Model file for the job. Use its own axes, mm. Round coordinates to 2 decimals unless told otherwise and drop trailing zeros. Loops run counter-clockwise (first coordinate to the right, second up) from the corner with the lowest first, then second, coordinate; pieces in that order, holes last.
from build123d import *

# Parameters (mm, degrees)
BOSS_EXTRU_1_DEPTH = 52
CONG_1_R           = 2
ESQUISSE3_R        = 1
BOSS_EXTRU_2_DEPTH = 40


with BuildPart() as part:
    # Esquisse2 → Boss.-Extru.1 (new body)
    with BuildSketch(Plane.XY):
        with BuildLine():
            ThreePointArc((6, 7.348469228), (0, 6.742346142), (-6, 7.348469228))
            ThreePointArc((-6, 7.348469228), (-15, 0), (-6, -7.348469228))
            ThreePointArc((-6, -7.348469228), (0, -6.742346142), (6, -7.348469228))
            ThreePointArc((6, -7.348469228), (0, 0), (6, 7.348469228))
        make_face()
        with BuildLine():
            ThreePointArc((9, 7.348469228), (7.5, 7.5), (6, 7.348469228))
            ThreePointArc((6, 7.348469228), (0, 0), (6, -7.348469228))
            ThreePointArc((6, -7.348469228), (7.5, -7.5), (9, -7.348469228))
            ThreePointArc((9, -7.348469228), (13.309475024, -4.743416484), (15, 1.6e-08))
            ThreePointArc((15, 1.6e-08), (13.309475014, 4.743416497), (9, 7.348469228))
        make_face()
        with BuildLine():
            ThreePointArc((21, 7.348469228), (15, 6.742346142), (9, 7.348469228))
            ThreePointArc((9, 7.348469228), (13.309475014, 4.743416497), (15, 1.6e-08))
            ThreePointArc((15, 1.6e-08), (16.690524986, 4.743416497), (21, 7.348469228))
        make_face()
        with BuildLine():
            ThreePointArc((15, 1.6e-08), (13.309475024, -4.743416484), (9, -7.348469228))
            ThreePointArc((9, -7.348469228), (15, -6.742346142), (21, -7.348469228))
            ThreePointArc((21, -7.348469228), (16.690524976, -4.743416484), (15, 1.6e-08))
        make_face()
        with BuildLine():
            ThreePointArc((21, 7.348469228), (16.690524986, 4.743416497), (15, 1.6e-08))
            ThreePointArc((15, 1.6e-08), (16.690524976, -4.743416484), (21, -7.348469228))
            ThreePointArc((21, -7.348469228), (22.5, -7.5), (24, -7.348469228))
            ThreePointArc((24, -7.348469228), (28.309475025, -4.743416484), (30, 1.7e-08))
            ThreePointArc((30, 1.7e-08), (28.309475014, 4.743416497), (24, 7.348469228))
            ThreePointArc((24, 7.348469228), (22.5, 7.5), (21, 7.348469228))
        make_face()
        with BuildLine():
            ThreePointArc((36, 7.348469228), (30, 6.742346142), (24, 7.348469228))
            ThreePointArc((24, 7.348469228), (28.309475014, 4.743416497), (30, 1.7e-08))
            ThreePointArc((30, 1.7e-08), (31.690524986, 4.743416497), (36, 7.348469228))
        make_face()
        with BuildLine():
            ThreePointArc((30, 1.7e-08), (28.309475025, -4.743416484), (24, -7.348469228))
            ThreePointArc((24, -7.348469228), (30, -6.742346142), (36, -7.348469228))
            ThreePointArc((36, -7.348469228), (31.690524975, -4.743416484), (30, 1.7e-08))
        make_face()
        with BuildLine():
            ThreePointArc((36, 7.348469228), (31.690524986, 4.743416497), (30, 1.7e-08))
            ThreePointArc((30, 1.7e-08), (31.690524975, -4.743416484), (36, -7.348469228))
            ThreePointArc((36, -7.348469228), (37.5, -7.5), (39, -7.348469228))
            ThreePointArc((39, -7.348469228), (43.309475006, -4.743416507), (45, -4.3e-08))
            ThreePointArc((45, -4.3e-08), (43.309475033, 4.743416474), (39, 7.348469228))
            ThreePointArc((39, 7.348469228), (37.5, 7.5), (36, 7.348469228))
        make_face()
        with BuildLine():
            ThreePointArc((51, 7.348469228), (45, 6.742346142), (39, 7.348469228))
            ThreePointArc((39, 7.348469228), (43.309475033, 4.743416474), (45, -4.3e-08))
            ThreePointArc((45, -4.3e-08), (46.690524967, 4.743416474), (51, 7.348469228))
        make_face()
        with BuildLine():
            ThreePointArc((45, -4.3e-08), (43.309475006, -4.743416507), (39, -7.348469228))
            ThreePointArc((39, -7.348469228), (45, -6.742346142), (51, -7.348469228))
            ThreePointArc((51, -7.348469228), (46.690524994, -4.743416507), (45, -4.3e-08))
        make_face()
        with BuildLine():
            ThreePointArc((51, 7.348469228), (46.690524967, 4.743416474), (45, -4.3e-08))
            ThreePointArc((45, -4.3e-08), (46.690524994, -4.743416507), (51, -7.348469228))
            ThreePointArc((51, -7.348469228), (52.5, -7.5), (54, -7.348469228))
            ThreePointArc((54, -7.348469228), (60, 0), (54, 7.348469228))
            ThreePointArc((54, 7.348469228), (52.5, 7.5), (51, 7.348469228))
        make_face()
        with BuildLine():
            ThreePointArc((66, 7.348469228), (60, 6.742346142), (54, 7.348469228))
            ThreePointArc((54, 7.348469228), (60, 0), (54, -7.348469228))
            ThreePointArc((54, -7.348469228), (60, -6.742346142), (66, -7.348469228))
            ThreePointArc((66, -7.348469228), (75, 0), (66, 7.348469228))
        make_face()
    extrude(amount=BOSS_EXTRU_1_DEPTH)

    # Congé1
    cong_1_edges = [part.edges().sort_by_distance(p)[0] for p in [
        (7.5, -7.5, 52),
        (-15, 0, 52),
        (15, -6.742346142, 52),
        (22.5, -7.5, 52),
        (-15, 0, 0),
        (0, 6.742346142, 0),
        (7.5, 7.5, 0),
        (15, 6.742346142, 0),
        (22.5, 7.5, 0),
        (30, 6.742346142, 0),
        (37.5, 7.5, 0),
        (45, 6.742346142, 0),
        (52.5, 7.5, 0),
        (60, 6.742346142, 0),
        (30, -6.742346142, 52),
        (75, 0, 0),
        (60, -6.742346142, 0),
        (52.5, -7.5, 0),
        (45, -6.742346142, 0),
        (37.5, -7.5, 0),
        (30, -6.742346142, 0),
        (22.5, -7.5, 0),
        (15, -6.742346142, 0),
        (7.5, -7.5, 0),
        (0, -6.742346142, 0),
        (37.5, -7.5, 52),
        (45, -6.742346142, 52),
        (52.5, -7.5, 52),
        (60, -6.742346142, 52),
        (0, -6.742346142, 52),
        (75, 0, 52),
        (60, 6.742346142, 52),
        (52.5, 7.5, 52),
        (45, 6.742346142, 52),
        (37.5, 7.5, 52),
        (30, 6.742346142, 52),
        (22.5, 7.5, 52),
        (15, 6.742346142, 52),
        (7.5, 7.5, 52),
        (0, 6.742346142, 52),
    ]]
    fillet(cong_1_edges, radius=CONG_1_R)

    # Esquisse3 → Boss.-Extru.2 (add)
    with BuildSketch(Plane(origin=(0, 0, 0), x_dir=(0, 0, -1), z_dir=(1, 0, 0))):
        with Locations((-50.5, 1.25)):
            Circle(ESQUISSE3_R)
        with Locations((-50.5, -1.25)):
            Circle(ESQUISSE3_R)
    extrude(amount=-BOSS_EXTRU_2_DEPTH)


solid = part.part
Q1. Pull direction Y, two halves, no side cores. Call faces 1 (the face through (-15, 0, 26)), 2 (the face through (-26.914, 1.55, 49.546)), 3 (the face through (30.085, 6.742, 25.664)), 4 (the face through (-26.914, -0.95, 49.546)): pulls with the +Y half, pulls with the -Y half, needs draft (parallel to the pull), parting line crosses it, or undercut.
Q2. Slice it at B-B on z = 25. Give the cut face in (x, y).
Q3. Flat gauge pins, fed straight in: P1, Ø2, axis at y = 5.5, z = 26.5, coming from the +X side; P2, Ø1, axis at y = 2.5, z = 43.5, coming from the -X side; P3, Ø1, axis at x = 1, z = 30.5, coming from the +Y side. Where does each tip first touch, or does it go through?
Q4. Slice it at A-A on x = -28. Give the cut face in (y, z).
Q5. Probe line 1 (Y direction, x = 53, z = 22.5); line 2 (Y direction, x = 1, z = 30); line 3 (X direction, y = -1.75, z = 24.5). List the from-to ranges inside material, lowest first.
Reply:
1. face 1: parting line crosses it
1. face 2: undercut
1. face 3: pulls with the +Y half
1. face 4: undercut
2. outline: (-6, -7.35) arc R30 cw to (6, -7.35) arc R7.5 ccw to (9, -7.35) arc R30 cw to (21, -7.35) arc R7.5 ccw to (24, -7.35) arc R30 cw to (36, -7.35) arc R7.5 ccw to (39, -7.35) arc R30 cw to (51, -7.35) arc R7.5 ccw to (54, -7.35) arc R30 cw to (66, -7.35) arc R7.5 ccw (long way) to (66, 7.35) arc R30 cw to (54, 7.35) arc R7.5 ccw to (51, 7.35) arc R30 cw to (39, 7.35) arc R7.5 ccw to (36, 7.35) arc R30 cw to (24, 7.35) arc R7.5 ccw to (21, 7.35) arc R30 cw to (9, 7.35) arc R7.5 ccw to (6, 7.35) arc R30 cw to (-6, 7.35) arc R7.5 ccw (long way) to start
3. P1: stops at x = 73.5
3. P2: stops at x = -14.73
3. P3: stops at y = 6.78
4. outline: circle Ø2 at (-1.25, 50.5); circle Ø2 at (1.25, 50.5)
5. line 1: y = -7.48 to 7.48
5. line 2: y = -6.76 to 6.76
5. line 3: x = -14.79 to 74.79
